Autodesk Inventor part; units mm, degrees
ref_plane "YZ Plane" through (0, 0, 0) normal (1, 0, 0) x (0, 1, 0)
ref_plane "XZ Plane" through (0, 0, 0) normal (0, 1, 0) x (-1, 0, 0)
ref_plane "XY Plane" through (0, 0, 0) normal (0, 0, 1) x (1, 0, 0)
sketch "Boceto1" plane through (0, 0, 0) normal (0, 1, 0) x (-1, 0, 0)
  circle A0 centre (0, 0) radius 75
  circle A1 centre (0, 0) radius 62.5
  circle A2 centre (62.5, 0) radius 5
  circle A3 centre (0, 0) radius 13
  circle A4 centre (0, 0) radius 12
  circle A5 centre (-47.25, 15.2) radius 1.5
  circle A6 centre (-47.25, -10.8) radius 1.5
  circle A7 centre (-31.25, 54.1266) radius 5
  circle A8 centre (-31.25, -54.1266) radius 5
extrude "Extrusión1" add sketch "Boceto1" along normal blind 14 contours A0 | A2 A1 A8 A7
extrude "Extrusión2" add sketch "Boceto1" along normal blind 8 contours A3
thread "Rosca1"
thread "Rosca2"
thread "Rosca3"
thread "Rosca4"
thread "Rosca5"
properties part number "1.1.1.Base Sta.Plate"
Source: CAD feature listing. Evaluate the final solid. Frame: model axes, mm. A direction names the side the tool comes from. Give positions to 0.01 mm unless a question says otherwise; leave off trailing zeros. Loops run counter-clockwise (first coordinate to the right, second up) from the corner with the lowest first, then second, coordinate; pieces in that order, holes last. Notation, with made-up numbers: (57.5, 3.25) - (89.5, 3.25) arc R30 ccw to (89.5, 37.25) - close; hole circle Ø4 at (8.25, 31.5). An arc over 180 degrees is marked (long way). Use CSV: the item, a comma, the result in double quotes. Start each with the question number.
1. Section C-C (y = 3.75). Output: boundary loops of the cut face in (x, z), then the cut area to 3 significant figures.
2. Ray query, L1, parallel to Z at x = 31.25, y = 9.5; L2, parallel to Z at x = 47.25, y = 10.25; L3, parallel to X at y = 5.25, z = -53.5. Return the intervals inside material, ascending.
3. Section D-D (x = 30.5). Output: boundary loops of the cut face in (y, z), then the cut area to 3 significant figures.
4. Pin query (flat end, axial travel): pin 1 (1.8 mm diameter, centred on x = 47.25, z = -10.8, fed in from +Y); pin 2 (6 mm diameter, centred on y = 2, z = -59.5, fed in from -X); pin 3 (6 mm diameter, centred on x = -49, y = 11.5, fed in from -Z); pin 4 (5 mm diameter, centred on x = 24.5, y = 10, fed in from +Z). Return the tip coordinate at first contact, or that it passes through.
5. Draft query along X for faces 3 (the cylindrical face through (32.334, 6.902, -49.245)), 4 (the cylindrical face through (9.764, 6.902, -74.362)), 5 (the flat face through (1, 0, -16)). Return one class per face: +X half, -X half, draft (parallel to the pull), parting line (faces both ways), or undercut.
6. Reachability of faces 1 (the flat face through (-9, 8, -9)), 2 (the flat face through (1, 14, -16)) from +Z, -Z, +X, -X, +Y, -Y: full face, straight path, thin tool, end or side. Return the list, or none.
7. Section B-B (z = 0). Output: boundary loops of the cut face in (x, y).
8. Section A-A (x = 0). Output: boundary loops of the cut face in (y, z), then the cut area to 3 significant figures.
Response:
1,outline,"circle Ø150 at (0, 0); hole circle Ø10 at (-62.5, 0); hole circle Ø24 at (0, 0); hole circle Ø10 at (31.25, -54.13); hole circle Ø10 at (31.25, 54.13); hole circle Ø3 at (47.25, -10.8); hole circle Ø3 at (47.25, 15.2)"
1,area,"17,000 mm²"
2,L1,"-68.18 to -59.13, -49.13 to 49.13, 59.13 to 68.18"
2,L2,"-58.24 to -12.3, -9.3 to 13.7, 16.7 to 58.24"
2,L3,"-52.56 to 26.29, 36.21 to 52.56"
3,outline,"(0, -68.52) - (14, -68.52) - (14, -59.07) - (0, -59.07) - close; (0, -49.18) - (14, -49.18) - (14, 49.18) - (0, 49.18) - close; (0, 59.07) - (14, 59.07) - (14, 68.52) - (0, 68.52) - close"
3,area,"1,640 mm²"
4,pin 1,"through"
4,pin 2,"x = -49.32"
4,pin 3,"z = -59.24"
4,pin 4,"z = 71.7"
5,face 3,"undercut"
5,face 4,"parting line"
5,face 5,"draft"
6,face 1,"+Y"
6,face 2,"+Z, -Z, +X, -X, +Y"
7,outline,"(-75, 0) - (-67.5, 0) - (-67.5, 14) - (-75, 14) - close; (-57.5, 0) - (-12, 0) - (-12, 8) - (-13, 8) - (-13, 14) - (-57.5, 14) - close; (12, 0) - (75, 0) - (75, 14) - (13, 14) - (13, 8) - (12, 8) - close"
8,outline,"(0, -75) - (14, -75) - (14, -13) - (8, -13) - (8, -12) - (0, -12) - close; (0, 12) - (8, 12) - (8, 13) - (14, 13) - (14, 75) - (0, 75) - close"
8,area,"1,750 mm²"
